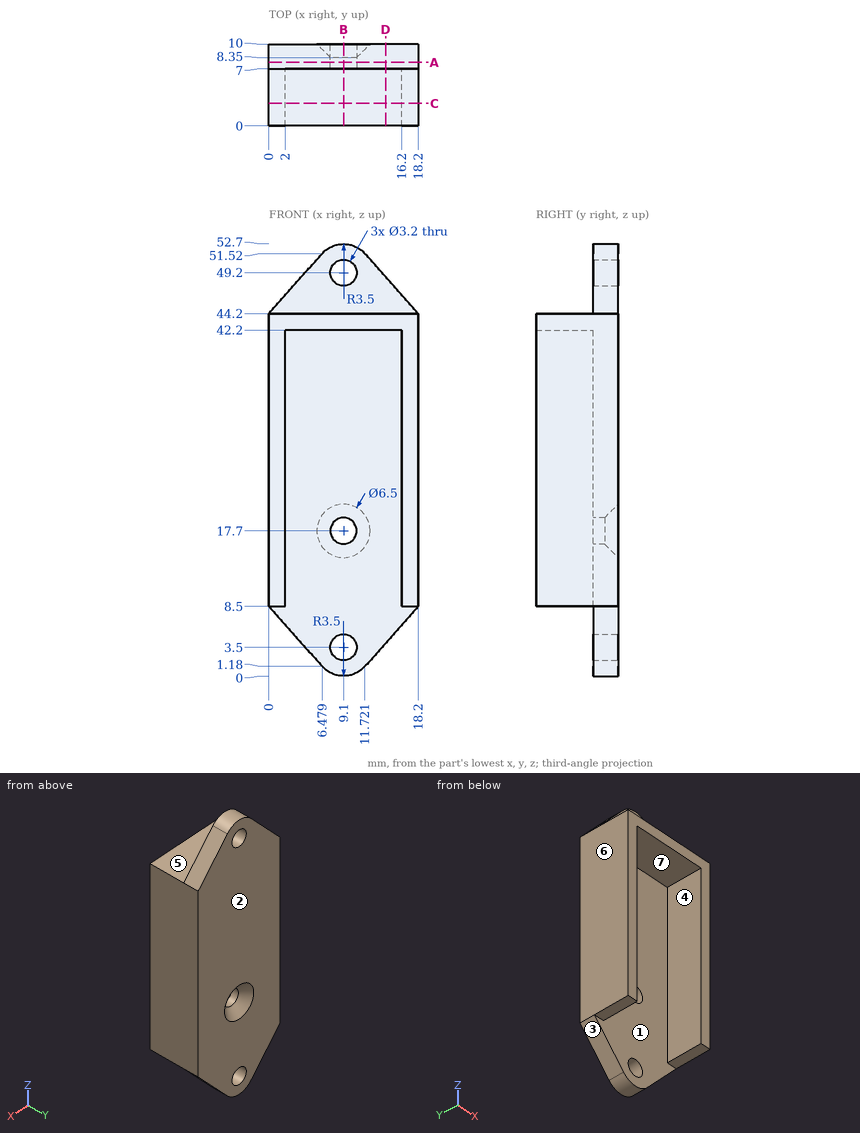
Answer from the drawing. Dimensions are ordinates in mm from the lowest x, y and z of the part. A direction names the side the tool comes from. Coordinates: 2 decimals unless noted, no trailing zeros. Write each loop counter-clockwise with the first axis right and the second up, starting at its lowest first coordinate (ties: lowest second). Pieces come first, ordered by that corner, then holes. Notation, with made-up numbers: (-31.75, -38) - (-18.75, -38) arc R19 ccw to (-18.75, -24) - close; hole circle Ø5 at (27, 4). An arc over 180 degrees is marked (long way). Return JSON: item names as keys, results as strings. Group by question number.
Q1. The part is cut by section D-D on x = 14.25. Write down the section's boundary in (y, z), and give its area (3 significant figures).
Q2. For a pull along X with two mould halves and no side action, classify the marked faces 1, 2, 3 and 4 as +X half, -X half, draft (parallel to the pull), parting line (faces both ways), or undercut.
Q3. The part is cut by section C-C on y = 2.75. Write down the section's boundary in (x, z).
Q4. The part is cut by section A-A on y = 7.75. Write down the section's boundary in (x, z), and give its area (3 significant figures).
Q5. Find the intervals of material crossed by line 1 along Z through (x, y) = (9.1, 7.9); line 2 along X through (y, z) = (6.75, 28); line 3 along Z through (x, y) = (9.1, 9.25), in increasing order. Write a range as [from, to].
Q6. Which of the six approach directions +Z, -Z, +X, -X, +Y, -Y give full straight-line access (tool end or side, diameter ignored) to the marked faces 5, 6 and 7?
Q7. Flat-ended cylindrical pins translate along their axes: pin 1 Ø3 at (x, y) = (4.5, 3.5) entering from -Z; pin 2 Ø2.5 at (x, z) = (9.1, 17.7) entering from -Y; pin 3 Ø10 at (x, z) = (3, 46) entering from -Y; pin 4 Ø5 at (x, z) = (9.1, 3.5) entering from -Y. Find the tip coordinate at first contact, or state that the pin passes through.
Q8. The part is cut by section B-B on x = 9.1. Write down the section's boundary in (y, z), and give its area (3 significant figures).
Evaluation:
{
 "1": {"outline": "(0, 42.2) - (7, 42.2) - (7, 4.04) - (10, 4.04) - (10, 48.66) - (7, 48.66) - (7, 44.2) - (0, 44.2) - close", "area": "148 mm2"},
 "2": {"face 1": "undercut", "face 2": "draft", "face 3": "-X half", "face 4": "undercut"},
 "3": {"outline": "(0, 8.5) - (2, 8.5) - (2, 42.2) - (16.2, 42.2) - (16.2, 8.5) - (18.2, 8.5) - (18.2, 44.2) - (0, 44.2) - close"},
 "4": {"outline": "(0, 8.5) - (6.48, 1.18) arc R3.5 ccw to (11.72, 1.18) - (18.2, 8.5) - (18.2, 44.2) - (11.72, 51.52) arc R3.5 ccw to (6.48, 51.52) - (0, 44.2) - close; hole circle Ø3.2 at (9.1, 3.5); hole circle Ø3.2 at (9.1, 17.7); hole circle Ø3.2 at (9.1, 49.2)", "area": "806 mm2"},
 "5": {"line 1": "z = [0, 1.9], [5.1, 16.1], [19.3, 47.6], [50.8, 52.7]", "line 2": "x = [0, 2], [16.2, 18.2]", "line 3": "z = [0, 1.9], [5.1, 15.2], [20.2, 47.6], [50.8, 52.7]"},
 "6": {"face 5": "+Z, +X, -X, -Y", "face 6": "+Z, -Z, -X, +Y, -Y", "face 7": "-Z, -Y"},
 "7": {"pin 1": "stops at z = 42.2", "pin 2": "passes through", "pin 3": "stops at y = 0", "pin 4": "stops at y = 7"},
 "8": {"outline": "(0, 42.2) - (7, 42.2) - (7, 19.3) - (8.35, 19.3) - (10, 20.95) - (10, 47.6) - (7, 47.6) - (7, 44.2) - (0, 44.2) - close; (7, 0) - (10, 0) - (10, 1.9) - (7, 1.9) - close; (7, 5.1) - (10, 5.1) - (10, 14.45) - (8.35, 16.1) - (7, 16.1) - close; (7, 50.8) - (10, 50.8) - (10, 52.7) - (7, 52.7) - close", "area": "141 mm2"}
}
